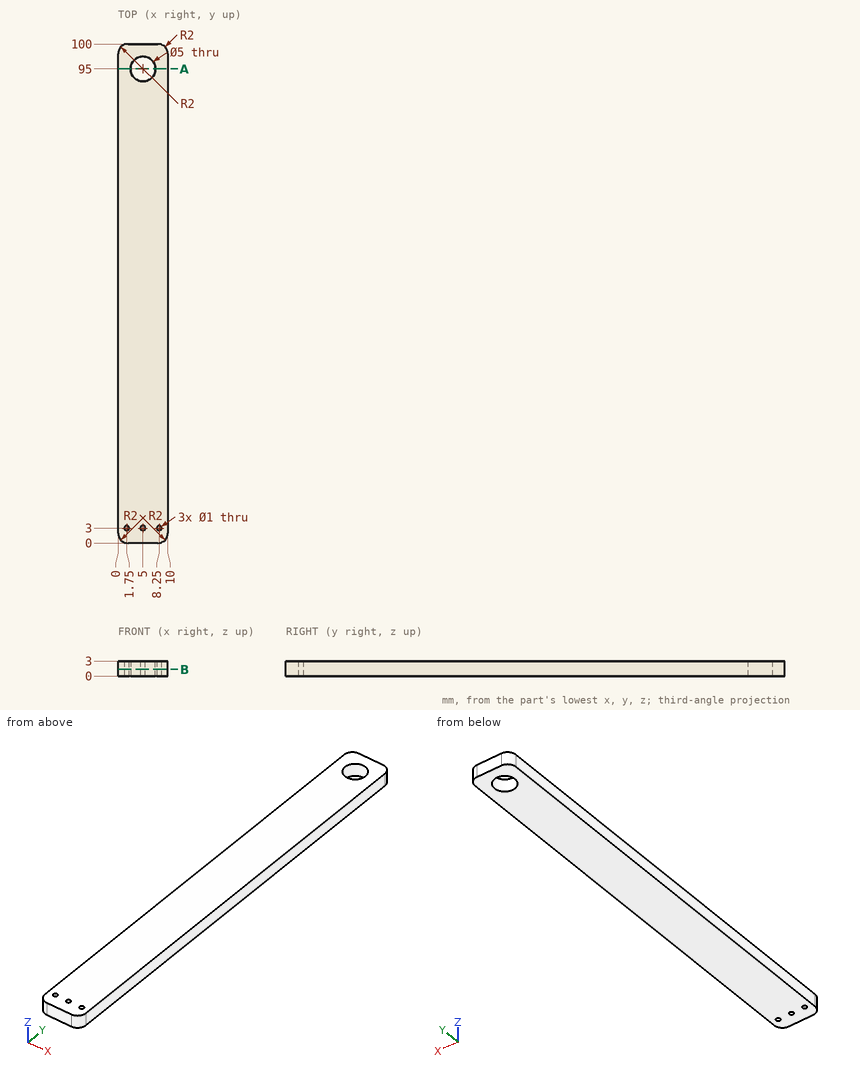
Here's the drawing with two shaded views (mm, measured from the low corner). I have some questions. Round coordinates to 2 decimals unless told otherwise and drop trailing zeros. Loops run counter-clockwise (first coordinate to the right, second up) from the corner with the lowest first, then second, coordinate; pieces in that order, holes last. Notation, with made-up numbers: (70.5, 88) - (92.5, 88) arc R33 ccw to (92.5, 118) - close; hole circle Ø1 at (74.25, -19.75). An arc over 180 degrees is marked (long way). Use CSV: the item, a comma, the result in double quotes.
Item 1: I need wall thicknesses on L1, parallel to Y at x = 5, z = 1.8; L2, parallel to X at y = 95, z = 1.3; L3, parallel to Y at x = 1.75, z = 2.7. Which ranges of each line are inside material? Lowest first, please. Write a range as [from, to].
Here are the results:
L1,"y = [0, 2.5], [3.5, 92.5], [97.5, 100]"
L2,"x = [0, 2.5], [7.5, 10]"
L3,"y = [0.02, 2.5], [3.5, 99.98]"
Item 2: If we section it at A-A on y = 95: List the corners of the cut face in (x, z) for me, then the cut area to 3 significant figures.
Here are the results:
outline,"(0, 0) - (2.5, 0) - (2.5, 3) - (0, 3) - close; (7.5, 0) - (10, 0) - (10, 3) - (7.5, 3) - close"
area,"15.0 mm²"
Item 3: If we section it at B-B on z = 1.35: List the corners of the cut face in (x, y) for me.
Here are the results:
outline,"(0, 2) arc R2 ccw to (2, 0) - (8, 0) arc R2 ccw to (10, 2) - (10, 98) arc R2 ccw to (8, 100) - (2, 100) arc R2 ccw to (0, 98) - close; hole circle Ø1 at (1.75, 3); hole circle Ø5 at (5, 95); hole circle Ø1 at (5, 3); hole circle Ø1 at (8.25, 3)"
